from build123d import *

# Parameters (mm, degrees)
F0_W     = 32
F0_H     = 16
F0_R     = 2.5
F1_DEPTH = 3
F2_W     = 32
F2_H     = 3
F3_DEPTH = 7
F5_DEPTH = 32
F6_R     = 2.5
F7_DEPTH = 3


with BuildPart() as f1:
    # F0 (on Top) → F1 (new body)
    with BuildSketch(Plane.XY):
        Rectangle(F0_W, F0_H)
        with Locations((-8, -2)):
            Circle(F0_R, mode=Mode.SUBTRACT)
        with Locations((8, -2)):
            Circle(F0_R, mode=Mode.SUBTRACT)
    extrude(amount=F1_DEPTH)

    # F2 (on face) → F3 (join)
    with BuildSketch(Plane.XY.offset(3)):
        with Locations((0, 6.5)):
            Rectangle(F2_W, F2_H)
    extrude(amount=F3_DEPTH)

    # F4 (on face) → F5 (join)
    with BuildSketch(Plane(origin=(-16, 0, 0), x_dir=(0, -1, 0), z_dir=(-1, 0, 0))):
        Polygon((-8, 10), (-8, 0), (-5, 0), (-5, 3), (-5, 10), align=None)
    extrude(amount=F5_DEPTH)

    # F6 (on face) → F7 (cut)
    with BuildSketch(Plane.XZ.offset(-5)):
        with Locations((-40, 4.5)):
            Circle(F6_R)
        with Locations((-24, 4.5)):
            Circle(F6_R)
    extrude(amount=-F7_DEPTH, mode=Mode.SUBTRACT)


solid = f1.part
Can you work these out from the model? Positions are in its coordinate system, mm. A direction names the side the tool comes from. Coordinates: 2 decimals unless noted, no trailing zeros. Loops run counter-clockwise (first coordinate to the right, second up) from the corner with the lowest first, then second, coordinate; pieces in that order, holes last. Notation, with made-up numbers: M -22,-13 L -10,-13 A20 cw -10,22 Z; hole C 22,30 d8. An arc over 180 degrees is marked long. Return JSON: item names as keys, results as strings. Group by question number.
Item 1: On a 3-axis mill with a long thin cutter (end or side, diameter ignored), from which of +Z, -Z, +X, -X, +Y, -Y can I reach the whole of each face in a straight line? I mean faces 1 (the flat face through (0, -1, 3)), 2 (the flat face through (-8, 2, 0)). Say none if no direction works.
Item 2: Imagine slicing it at A-A (y = -3.5). Please give me the cut outline in (x, z).
Item 3: I'm going to push flat-ended pins straight in: pin 1 Ø2 at (y, z) = (3.5, 8) entering from +X; pin 2 Ø2.5 at (y, z) = (-1.5, 2) entering from -X; pin 3 Ø8 at (x, y) = (8, -2) entering from +Z. Where does each tip first touch, or does it pass through?
Item 4: If I drill on L1, parallel to Z at x = -24, y = 6.25; L2, parallel to Y at x = -8, z = 2.2; L3, parallel to Y at x = -26.5, z = 6, over which ranges is the centre line in solid material (lowest first)? Write a range as from..to.
Item 5: Imagine slicing it at B-B (z = 4.5). Please give me the cut outline in (x, y).
Item 6: Imagine slicing it at C-C (x = -24). Please give me the cut outline in (y, z), and give its area (3 significant figures).
Item 7: Thinking about a two-plate mould opening in Z: for faces 3 (the flat face through (-16, -2, 1)), 4 (the cylindrical face through (-37.69, 6.48, 3.54)), 5 (the cylindrical face through (-26, 6, 6)), 6 (the flat face through (-16, 6, 10)), which applies, released by +Z, released by -Z, zero draft, split by the parting line, or undercut?
Item 8: Imagine slicing it at D-D (y = 6.5). Please give me the cut outline in (x, z).
Verdict:
{
 "1": {"face 1": "+Z, +X, -X, -Y", "face 2": "-Z, +X, -X, +Y, -Y"},
 "2": {"outline": "M -16,0 L -10,0 L -10,3 L -16,3 Z; M -6,0 L 6,0 L 6,3 L -6,3 Z; M 10,0 L 16,0 L 16,3 L 10,3 Z"},
 "3": {"pin 1": "passes through", "pin 2": "stops at x = -16", "pin 3": "stops at z = 3"},
 "4": {"L1": "z = 0..2, 7..10", "L2": "y = -8..-4.5, 0.5..8", "L3": "y = 5..8"},
 "5": {"outline": "M -48,5 L -42.5,5 L -42.5,8 L -48,8 Z; M -37.5,5 L -26.5,5 L -26.5,8 L -37.5,8 Z; M -21.5,5 L 16,5 L 16,8 L -21.5,8 Z"},
 "6": {"outline": "M 5,0 L 8,0 L 8,2 L 5,2 Z; M 5,7 L 8,7 L 8,10 L 5,10 Z", "area": "15.0 mm^2"},
 "7": {"face 3": "zero draft", "face 4": "undercut", "face 5": "undercut", "face 6": "released by +Z"},
 "8": {"outline": "M -48,0 L 16,0 L 16,10 L -48,10 Z; hole C -40,4.5 d5; hole C -24,4.5 d5"}
}
